Can you work these out from the drawing? Everything is in mm from the part's minimum corner. A direction names the side the tool comes from. Round coordinates to 2 decimals unless told otherwise and drop trailing zeros. Order: outer loops, then holes, each group sorted by start corner. A loop starts at its lowest first (then second) coordinate and runs counter-clockwise, first axis right, second up. Notation, with made-up numbers: M -40,23.5 L 15,23.5 A15 cw 15,38.5 Z; hole C 80.25,19 d8. An arc over 180 degrees is marked long. Write each question's results on one line, items separated by ' | '. Start each with the question number.
1. Please list where these lines run through material, in increasing order: L1, parallel to X at y = 24.5, z = 4; L2, parallel to Y at x = 6, z = 1.5; L3, parallel to Y at x = 3.5, z = 3.
2. Suppose I cut it at C-C on z = 6. Write out the boundary of the cut face in (x, y) (1 decimal).
3. Suppose I cut it at D-D on z = 8.75. Write out the boundary of the cut face in (x, y).
4. Suppose I cut it at A-A on x = 2.75. Write out the boundary of the cut face in (y, z) (1 decimal).
5. For the marked faces 1 and 2, which set-ups out of +Z, -Z, +X, -X, +Y, -Y let a thin tool reach every point of the face, with its end or its side?
6. We'd pull the mould along Y, two halves only. Please class the marked faces 3, 4 and 5: released by +Y, released by -Y, zero draft, split by the parting line, or undercut.
7. Suppose I cut it at B-B on y = 37. Write out the boundary of the cut face in (x, z), and give its area (3 significant figures).
8. I'm going to push flat-ended pins straight in: pin 1 (1.8 mm diameter, centred on x = 4.5, z = 6.5, fed in from +Y) (1 decimal); pin 2 (5 mm diameter, centred on x = 4, y = 33.5, fed in from -Z). Where does each tip first touch, or does it pass through?
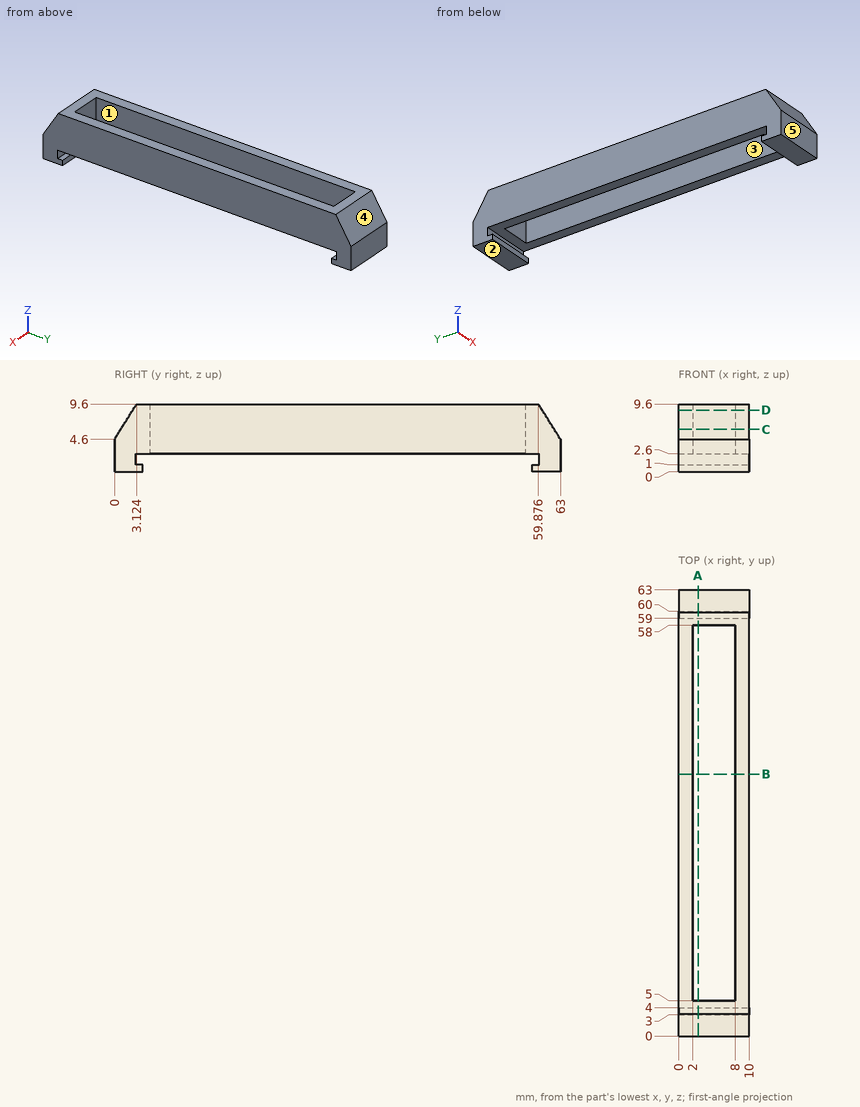
Filled sheet:
1) L1: x = 0 to 2, 8 to 10 | L2: y = 0 to 3, 60 to 63 | L3: y = 0 to 5, 58 to 63
2) outline: M 0,0.9 L 10,0.9 L 10,62.1 L 0,62.1 Z; hole M 2,5 L 8,5 L 8,58 L 2,58 Z
3) outline: M 0,2.59 L 10,2.59 L 10,60.41 L 0,60.41 Z; hole M 2,5 L 8,5 L 8,58 L 2,58 Z
4) outline: M 0,0 L 4,0 L 4,1 L 3,1 L 3,2.6 L 5,2.6 L 5,9.6 L 3.1,9.6 L 0,4.6 Z; M 58,2.6 L 60,2.6 L 60,1 L 59,1 L 59,0 L 63,0 L 63,4.6 L 59.9,9.6 L 58,9.6 Z
5) face 1: +Z, -Z | face 2: -Z, +X, -X, +Y, -Y
6) face 3: undercut | face 4: released by +Y | face 5: released by -Y
7) outline: M 0,2.6 L 2,2.6 L 2,9.6 L 0,9.6 Z; M 8,2.6 L 10,2.6 L 10,9.6 L 8,9.6 Z | area: 28.0 mm^2
8) pin 1: stops at y = 62.4 | pin 2: stops at z = 2.6
